Job drawing, mm, ordinate dimensions from the low corner. One solid piece. A direction names the side the tool comes from. Round coordinates to 2 decimals unless told otherwise and drop trailing zeros. Write each loop counter-clockwise with the first axis right and the second up, starting at its lowest first coordinate (ties: lowest second). Pieces come first, ordered by that corner, then holes. Notation, with made-up numbers: (-5.5, -38) -> (10.5, -38) arc R15 ccw to (10.5, -14) -> close; hole circle Ø6 at (52, 62.25). An arc over 180 degrees is marked (long way). Use CSV: the item, a comma, the result in double quotes. Start each with the question number.
(1) Probe line 1 (Z direction, x = 152.4, y = 86.5); line 2 (Z direction, x = 151.5, y = 36.5); line 3 (Y direction, x = 266.5, z = 100). List the from-to ranges inside material, lowest first. Write a range as [from, to].
(2) Two-plate mould, pull along Z, no slides. Class the marked faces 1, 2 and 3: released by +Z, released by -Z, zero draft, split by the parting line, or undercut.
(3) Saw through at C-C (y = 58.5). Give the cut face in (x, z), plus the area to 3 significant figures.
(4) Saw through at D-D (x = 58.5). Give the cut face in (y, z).
(5) Drop flat-ended pins along their axis: pin 1 (5 mm diameter, centred on x = 100.5, y = 37.5, fed in from -Z); pin 2 (6 mm diameter, centred on x = 223, y = 34.5, fed in from -Z); pin 3 (4 mm diameter, centred on y = 91, z = 56.5, fed in from +X). Give the stop position or say it passes through.
(6) Which spindle directions (+Z, -Z, +X, -X, +Y, -Y) get a long thin tool onto all of the face, cutting with end or side? Do the marked faces 4 and 5. Say none if no direction does.
(7) Saw through at A-A (z = 152.4). Give the cut face in (x, y), plus the area to 3 significant figures.
(8) Saw through at B-B (x = 152.4). Give the cut face in (y, z), plus the area to 3 significant figures.
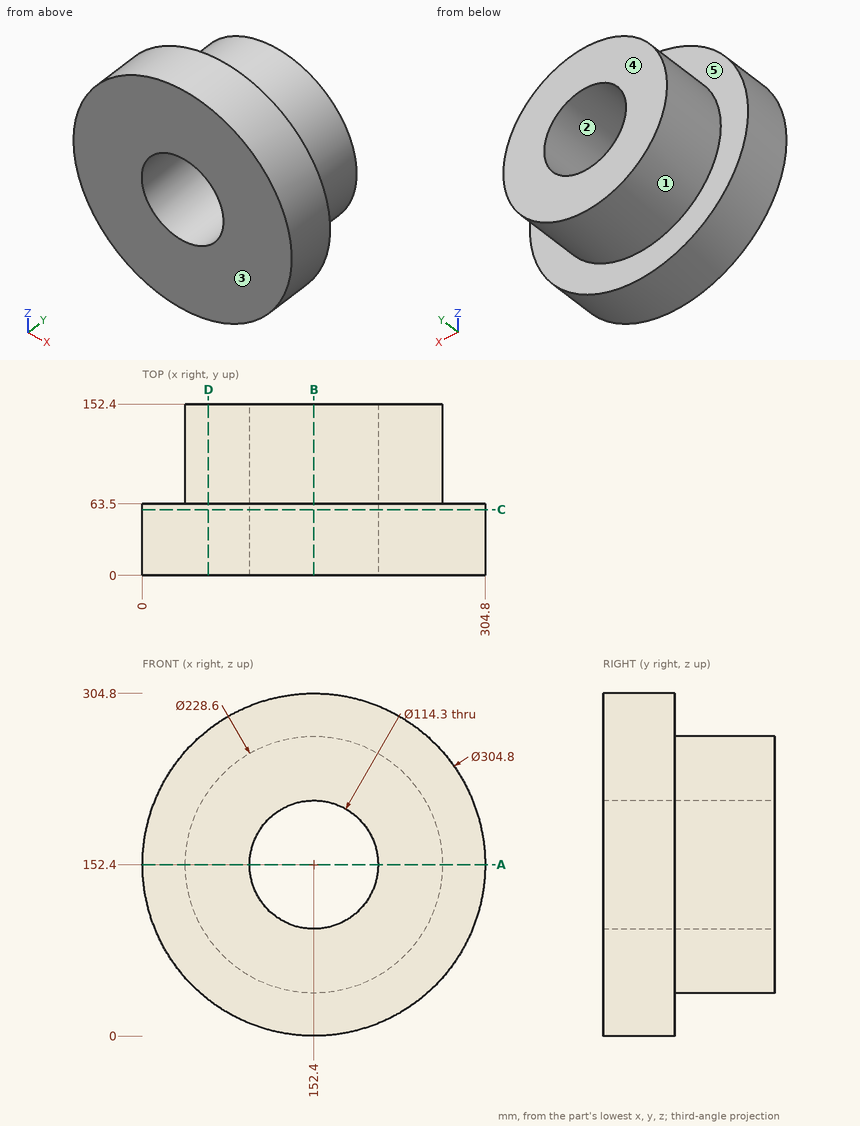
Answers:
1,line 1,"z = [38.1, 95.25], [209.55, 266.7]"
1,line 2,"z = [0, 95.26], [209.54, 304.8]"
1,line 3,"y = [0, 63.5]"
2,face 1,"split by the parting line"
2,face 2,"undercut"
2,face 3,"zero draft"
3,outline,"circle Ø304.8 at (152.4, 152.4); hole circle Ø114.3 at (152.4, 152.4)"
3,area,"62,700 mm²"
4,outline,"(0, 32.36) -> (63.5, 32.36) -> (63.5, 87.23) -> (152.4, 87.23) -> (152.4, 217.57) -> (63.5, 217.57) -> (63.5, 272.44) -> (0, 272.44) -> close"
5,pin 1,"stops at z = 8.23"
5,pin 2,"stops at z = 15.81"
5,pin 3,"stops at x = 217.57"
6,face 4,"+Z, -Z, +X, -X, +Y"
6,face 5,"+Y"
7,outline,"(0, 0) -> (95.25, 0) -> (95.25, 152.4) -> (38.1, 152.4) -> (38.1, 63.5) -> (0, 63.5) -> close; (209.55, 0) -> (304.8, 0) -> (304.8, 63.5) -> (266.7, 63.5) -> (266.7, 152.4) -> (209.55, 152.4) -> close"
7,area,"22,300 mm²"
8,outline,"(0, 0) -> (63.5, 0) -> (63.5, 38.1) -> (152.4, 38.1) -> (152.4, 95.25) -> (0, 95.25) -> close; (0, 209.55) -> (152.4, 209.55) -> (152.4, 266.7) -> (63.5, 266.7) -> (63.5, 304.8) -> (0, 304.8) -> close"
8,area,"22,300 mm²"
